Autodesk Inventor part; units mm, degrees
ref_plane "YZ Plane" through (0, 0, 0) normal (1, 0, 0) x (0, 1, 0)
ref_plane "XZ Plane" through (0, 0, 0) normal (0, 1, 0) x (-1, 0, 0)
ref_plane "XY Plane" through (0, 0, 0) normal (0, 0, 1) x (1, 0, 0)
sketch "Sketch1" plane through (0, 0, 0) normal (1, 0, 0) x (0, 1, 0)
  line L0 (-22.225, 9.525) -> (22.225, 9.525)
  line L1 (22.225, 9.525) -> (22.225, -9.525)
  line L2 (22.225, -9.525) -> (-22.225, -9.525)
  line L3 (-22.225, -9.525) -> (-22.225, 9.525)
  line L4 (-22.225, 9.525) -> (22.225, -9.525) construction
  line L5 (22.225, 9.525) -> (-22.225, -9.525) construction
  point P0 (0, 0)
  dimension "d0" = 44.45
  dimension "d1" = 19.05
extrude "Extrusion1" add sketch "Sketch1" along normal blind 12.7
sketch "Sketch2" plane through (12.7, 0, 0) normal (1, 0, 0) x (0, 0, -1)
  circle A0 centre (0, 12.7) radius 3.3782
  circle A1 centre (0, -12.7) radius 3.3782
  line L0 (-660.4, 0) -> (-660.4, 41.275)
  line L1 (-9.525, 22.225) -> (-9.525, -22.225)
  line L2 (-12.7, 22.225) -> (-12.7, -22.225)
  point P0 (0, 0)
  dimension "d4" = 3.175
  dimension "d5" = 12.7
hole "Hole1" at (12.7, 12.7, 0) at (12.7, -12.7, 0) direction (-1, 0, 0) diameter 4.9784 end through all
properties part number "Threaded Block" material "Aluminum 6061"
Build history of the part. All positions in model axes, mm. Round coordinates to 2 decimals unless told otherwise and drop trailing zeros. Write each loop counter-clockwise with the first axis right and the second up, starting at its lowest first coordinate (ties: lowest second). Pieces come first, ordered by that corner, then holes. Notation, with made-up numbers: M 49.5,35.5 L 101.5,35.5 A29 ccw 101.5,69.5 Z; hole C 25,-3 d10. An arc over 180 degrees is marked long. Answer in a Markdown table with one row per item.
1. Probe L1, parallel to Y at x = 10.25, z = 0 (3 decimals); L2, parallel to Z at x = 6.25, y = -12.7 (3 decimals); L3, parallel to Z at x = 1.5, y = -14 (3 decimals). List the from-to ranges inside material, lowest first. Write a range as [from, to].
Geometry check:
| item | result |
|---|---|
| L1 | [-22.225, -15.189], [-10.211, 10.211], [15.189, 22.225] |
| L2 | [-9.525, -2.489], [2.489, 9.525] |
| L3 | [-9.525, -2.123], [2.123, 9.525] |
2. Saw through at A-A (y = -12.7). List the corners of the cut face in (x, z) (3 decimals).
Geometry check:
| item | result |
|---|---|
| outline | M 0,-9.525 L 12.7,-9.525 L 12.7,-2.489 L 0,-2.489 Z; M 0,2.489 L 12.7,2.489 L 12.7,9.525 L 0,9.525 Z |
3. Mould opens along Z. For faces 1 (the face through (6.26, 10.6, -1.34)), 2 (the face through (6, 0, -9.525)), 3 (the face through (6.26, -15.17, 0.32)), 4 (the face through (6, 22.225, 0)) say: +Z half, -Z half, draft (parallel to the pull), parting line (faces both ways), or undercut.
Geometry check:
| item | result |
|---|---|
| face 1 | undercut |
| face 2 | -Z half |
| face 3 | undercut |
| face 4 | draft |
4. Saw through at B-B (x = 7.5). List the corners of the cut face in (y, z) (3 decimals).
Geometry check:
| item | result |
|---|---|
| outline | M -22.225,-9.525 L 22.225,-9.525 L 22.225,9.525 L -22.225,9.525 Z; hole C -12.7,0 d4.978; hole C 12.7,0 d4.978 |
5. Saw through at C-C (z = 0). List the corners of the cut face in (x, y) (3 decimals).
Geometry check:
| item | result |
|---|---|
| outline | M 0,-22.225 L 12.7,-22.225 L 12.7,-15.189 L 0,-15.189 Z; M 0,-10.211 L 12.7,-10.211 L 12.7,10.211 L 0,10.211 Z; M 0,15.189 L 12.7,15.189 L 12.7,22.225 L 0,22.225 Z |
